```python
from build123d import *

# Parameters (mm, degrees)
SKETCH1_R           = 7
SKETCH1_R_2         = 5
BOSS_EXTRUDE1_DEPTH = 12
SKETCH2_R           = 9
SKETCH2_R_2         = 7
SKETCH2_R_3         = 5
BOSS_EXTRUDE2_DEPTH = 2
FILLET1_R           = 0.3


with BuildPart() as part:
    # Sketch1 → Boss-Extrude1 (new body)
    with BuildSketch(Plane.XY):
        Circle(SKETCH1_R)
        Circle(SKETCH1_R_2, mode=Mode.SUBTRACT)
    extrude(amount=BOSS_EXTRUDE1_DEPTH)

    # Sketch2 → Boss-Extrude2 (add)
    # profile 1 of 2: a face of its own
    with BuildSketch(Plane.XY.offset(12)):
        Circle(SKETCH2_R)
        Circle(SKETCH2_R_2, mode=Mode.SUBTRACT)
    # profile 2 of 2: a face of its own
    with BuildSketch(Plane.XY.offset(12)):
        Circle(SKETCH2_R_2)
        Circle(SKETCH2_R_3, mode=Mode.SUBTRACT)
    extrude(amount=BOSS_EXTRUDE2_DEPTH)

    # Fillet1
    fillet1_edges = [part.edges().sort_by_distance(p)[0] for p in [
        (-9, 0, 12),
        (-9, 0, 14),
        (-7, 0, 0),
        (-7, 0, 12),
    ]]
    fillet(fillet1_edges, radius=FILLET1_R)


solid = part.part
```
The listing builds one solid part. Answer for the finished solid, in the listing's coordinates (mm). A direction names the side the tool comes from. Give positions to 0.01 mm unless a question says otherwise; leave off trailing zeros. Order: outer loops, then holes, each group sorted by start corner. A loop starts at its lowest first (then second) coordinate and runs counter-clockwise, first axis right, second up. Notation, with made-up numbers: (55.5, -34) -> (108.5, -34) arc R23 ccw to (108.5, 3) -> close; hole circle Ø11 at (71.25, 6.5). An arc over 180 degrees is marked (long way). Answer as CSV lines item,"result". Start each with the question number.
Q1. Given pin 1 (5 mm diameter, centred on x = -2.5, z = 7.5, fed in from -Y); pin 2 (6 mm diameter, centred on x = -7, z = 8.5, fed in from +Y); pin 3 (3 mm diameter, centred on x = 6.5, z = 9.5, fed in from -Y); pin 4 (2 mm diameter, centred on x = 1, y = 2, fed in from +Z), each flat-ended and moving along its own axis, determine where each tip first touches the part or whether it passes through.
Q2. A cutting plane is placed at A-A (x = 0). Determine the outline of the cut face in (y, z), then the cut area to 3 significant figures.
Q3. Find the intervals of material crossed by L1, parallel to Y at x = 0, z = 3.5; L2, parallel to X at y = -0.25, z = 4.5; L3, parallel to Z at x = -4.5, y = -7, in increasing order.
Q4. Determine the mould class of faces 3 (the cylindrical face through (-1.08, -4.88, 6.9)), 4 (the flat face through (4, -4, 14)), 5 (the cylindrical face through (6.466, -2.681, 5.92)) for opening direction X: pulls with the +X half, pulls with the -X half, needs draft (parallel to the pull), parting line crosses it, or undercut.
Q5. A cutting plane is placed at C-C (z = 9). Determine the outline of the cut face in (x, y).
Q6. Which of the six approach directions +Z, -Z, +X, -X, +Y, -Y give full straight-line access (tool end or side, diameter ignored) to faces 1 (the flat face through (-5, 6, 12)), 2 (the cylindrical face through (-1.172, 8.923, 12.99))?
Results found:
1,pin 1,"y = -7"
1,pin 2,"y = 5.74"
1,pin 3,"y = -4.9"
1,pin 4,"through"
2,outline,"(-9, 12.3) arc R0.3 ccw to (-8.7, 12) -> (-7.3, 12) arc R0.3 cw to (-7, 11.7) -> (-7, 0.3) arc R0.3 ccw to (-6.7, 0) -> (-5, 0) -> (-5, 14) -> (-8.7, 14) arc R0.3 ccw to (-9, 13.7) -> close; (5, 0) -> (6.7, 0) arc R0.3 ccw to (7, 0.3) -> (7, 11.7) arc R0.3 cw to (7.3, 12) -> (8.7, 12) arc R0.3 ccw to (9, 12.3) -> (9, 13.7) arc R0.3 ccw to (8.7, 14) -> (5, 14) -> close"
2,area,"63.9 mm2"
3,L1,"-7 to -5, 5 to 7"
3,L2,"-7 to -4.99, 4.99 to 7"
3,L3,"12 to 14"
4,face 3,"undercut"
4,face 4,"needs draft"
4,face 5,"parting line crosses it"
5,outline,"circle Ø14 at (0, 0); hole circle Ø10 at (0, 0)"
6,face 1,"-Z"
6,face 2,"+Z, -Z"
